Build history of the part. All positions in model axes, mm. Give positions to 0.01 mm unless a question says otherwise; leave off trailing zeros. Order: outer loops, then holes, each group sorted by start corner. A loop starts at its lowest first (then second) coordinate and runs counter-clockwise, first axis right, second up. Notation, with made-up numbers: (38.25, 54) - (63.25, 54) arc R10 cw to (63.25, 68) - close; hole circle Ø10 at (8.25, 38). An arc over 180 degrees is marked (long way). Use a Markdown table: item, result.
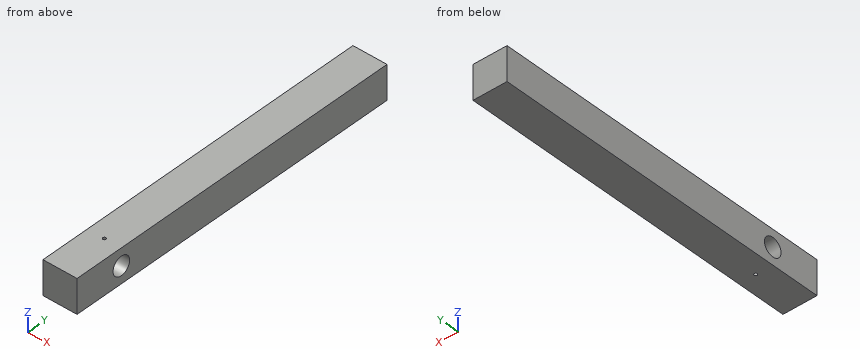
from build123d import *

# Parameters (mm, degrees)
F0_W     = 17.4625
F0_H     = 17.4625
F1_DEPTH = 177.8
F2_R     = 4.7625
F3_DEPTH = 17.4752
F4_R     = 0.79375
F5_DEPTH = 25.4


with BuildPart() as f1:
    # F0 (on Front) → F1 (new body)
    with BuildSketch(Plane.XZ):
        with Locations((-8.73125, 15.816035)):
            Rectangle(F0_W, F0_H)
    extrude(amount=F1_DEPTH)

    # F2 (on face) → F3 (cut)
    with BuildSketch(Plane(origin=(-17.4625, 0, 0), x_dir=(0, -1, 0), z_dir=(-1, 0, 0))):
        with Locations((152.4, 15.809685)):
            Circle(F2_R)
    extrude(amount=-F3_DEPTH, mode=Mode.SUBTRACT)

    # F4 (on face) → F5 (cut)
    with BuildSketch(Plane.XY.offset(24.547285)):
        with Locations((-8.73125, -152.4)):
            Circle(F4_R)
    extrude(amount=-F5_DEPTH, mode=Mode.SUBTRACT)


solid = f1.part
1) Pin check, flat tips, straight feed: P1, Ø4, axis at y = -93.5, z = 12, coming from the +X side; P2, Ø1.3, axis at x = -8.73, y = -152.4, coming from the -Z side. Stop position of each tip, or through.
Computed:
| item | result |
|---|---|
| P1 | stops at x = 0 |
| P2 | passes through |
2) Slice it at B-B (x = -11). Write the cut outline in (y, z) (1 decimal).
Computed:
| item | result |
|---|---|
| outline | (-177.8, 7.1) - (0, 7.1) - (0, 24.5) - (-177.8, 24.5) - close; hole circle Ø9.5 at (-152.4, 15.8) |
3) Slice it at A-A (z = 17.75). Write the cut outline in (x, y).
Computed:
| item | result |
|---|---|
| outline | (-17.46, -177.8) - (0, -177.8) - (0, -156.75) - (-17.46, -156.75) - close; (-17.46, -148.05) - (0, -148.05) - (0, 0) - (-17.46, 0) - close |
4) Wall check: line 1 (X direction, y = -152.4, z = 23.3) (1 decimal); line 2 (Z direction, x = -12.25, y = -152.4); line 3 (Y direction, x = -8.5, z = 14.75). Give the ranges that are in metal, low to high. Write a range as from..to.
Computed:
| item | result |
|---|---|
| line 1 | x = -17.5..-9.5, -7.9..0 |
| line 2 | z = 7.08..11.05, 20.57..24.55 |
| line 3 | y = -177.8..-157.04, -147.76..0 |
